Study the drawing (mm; zero at the part's minimum x, y, z) and answer. Round coordinates to 2 decimals unless told otherwise and drop trailing zeros. Write each loop counter-clockwise with the first axis right and the second up, starting at its lowest first coordinate (ties: lowest second). Pieces come first, ordered by that corner, then holes.
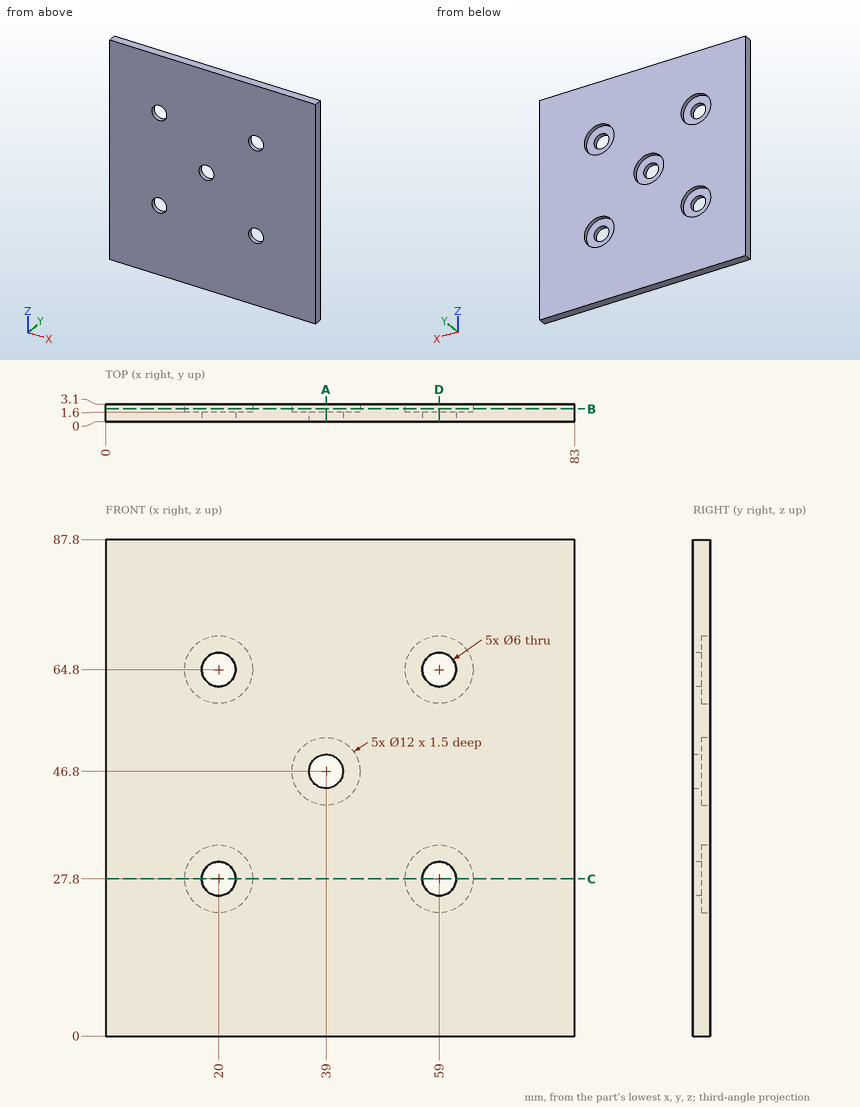
1. Section A-A on x = 39 is taken. Determine the outline of the cut face in (y, z), plus the area to 3 significant figures.
Geometry says:
outline: (0, 0) - (3.1, 0) - (3.1, 40.8) - (1.6, 40.8) - (1.6, 43.8) - (0, 43.8) - close; (0, 49.8) - (1.6, 49.8) - (1.6, 52.8) - (3.1, 52.8) - (3.1, 87.8) - (0, 87.8) - close
area: 245 mm2
2. Section C-C on z = 27.8 is taken. Determine the outline of the cut face in (x, y), plus the area to 3 significant figures.
Geometry says:
outline: (0, 0) - (17, 0) - (17, 1.6) - (14, 1.6) - (14, 3.1) - (0, 3.1) - close; (23, 0) - (56, 0) - (56, 1.6) - (53, 1.6) - (53, 3.1) - (26, 3.1) - (26, 1.6) - (23, 1.6) - close; (62, 0) - (83, 0) - (83, 3.1) - (65, 3.1) - (65, 1.6) - (62, 1.6) - close
area: 202 mm2
3. Straight lines are drawn through the part: line 1 along X through (y, z) = (1.1, 27.8); line 2 along Z through (x, y) = (20, 2.2); line 3 along Z through (x, y) = (64, 1.8). For each, find the intervals that lie inside material, in ascending order.
Geometry says:
line 1: x = 0 to 17, 23 to 56, 62 to 83
line 2: z = 0 to 21.8, 33.8 to 58.8, 70.8 to 87.8
line 3: z = 0 to 24.48, 31.12 to 61.48, 68.12 to 87.8
4. Section D-D on x = 59 is taken. Determine the outline of the cut face in (y, z), plus the area to 3 significant figures.
Geometry says:
outline: (0, 0) - (3.1, 0) - (3.1, 21.8) - (1.6, 21.8) - (1.6, 24.8) - (0, 24.8) - close; (0, 30.8) - (1.6, 30.8) - (1.6, 33.8) - (3.1, 33.8) - (3.1, 58.8) - (1.6, 58.8) - (1.6, 61.8) - (0, 61.8) - close; (0, 67.8) - (1.6, 67.8) - (1.6, 70.8) - (3.1, 70.8) - (3.1, 87.8) - (0, 87.8) - close
area: 217 mm2
5. Section B-B on y = 2.25 is taken. Determine the outline of the cut face in (x, z).
Geometry says:
outline: (0, 0) - (83, 0) - (83, 87.8) - (0, 87.8) - close; hole circle Ø12 at (20, 27.8); hole circle Ø12 at (20, 64.8); hole circle Ø12 at (39, 46.8); hole circle Ø12 at (59, 27.8); hole circle Ø12 at (59, 64.8)
6. Given pin 1 (9.5 mm diameter, centred on x = 23, z = 65, fed in from +Y); pin 2 (3.5 mm diameter, centred on x = 58.5, z = 25, fed in from +Y), each flat-ended and moving along its own axis, determine where each tip first touches the part or whether it passes through.
Geometry says:
pin 1: stops at y = 3.1
pin 2: stops at y = 1.6
